from build123d import *

# Parameters (mm, degrees)
F1_DEPTH = 7.9375
F2_R     = 1.98374
F3_R     = 3.69316
F4_R     = 1.35255
F5_DEPTH = 134.38632
F6_W     = 127
F6_H     = 1.70942
F7_DEPTH = 3.175
F8_R     = 1.35255
F9_DEPTH = 1.70942
F10_R    = 0.762


with BuildPart() as f1:
    # F0 (on Top) → F1 (new body)
    with BuildSketch(Plane.XY):
        Polygon((0, 30.55874), (0, 0), (-130.96748, 0), (-130.96748, 30.55874), (-132.6769, 30.55874), (-132.6769, -1.70942), (1.70942, -1.70942), (1.70942, 30.55874), align=None)
    extrude(amount=F1_DEPTH)

    # F2
    f2_edges = [f1.edges().sort_by_distance(p)[0] for p in [
        (0, 0, 3.96875),
        (-130.96748, 0, 3.96875),
    ]]
    fillet(f2_edges, radius=F2_R)

    # F3
    f3_edges = [f1.edges().sort_by_distance(p)[0] for p in [
        (1.70942, -1.70942, 3.96875),
        (-132.6769, -1.70942, 3.96875),
    ]]
    fillet(f3_edges, radius=F3_R)

    # F4 (on face) → F5 (cut, through all)
    with BuildSketch(Plane(origin=(-132.6769, 0, 0), x_dir=(0, -1, 0), z_dir=(-1, 0, 0))):
        with Locations((-26.58999, 3.96875)):
            Circle(F4_R)
        with Locations((-5.95249, 3.96875)):
            Circle(F4_R)
    extrude(amount=-F5_DEPTH, mode=Mode.SUBTRACT)

    # F6 (on face) → F7 (join)
    with BuildSketch(Plane(origin=(0, 0, 0), x_dir=(1, 0, 0), z_dir=(0, 0, -1))):
        with Locations((-65.48374, 0.85471)):
            Rectangle(F6_W, F6_H)
    extrude(amount=F7_DEPTH)

    # F8 (on face) → F9 (cut, through all)
    with BuildSketch(Plane.XZ.offset(1.70942)):
        with Locations((-125.01499, 0.79375)):
            Circle(F8_R)
        with Locations((-65.48374, 0.79375)):
            Circle(F8_R)
        with Locations((-5.95249, 0.79375)):
            Circle(F8_R)
    extrude(amount=-F9_DEPTH, mode=Mode.SUBTRACT)

    # F10
    f10_edges = [f1.edges().sort_by_distance(p)[0] for p in [
        (0.85471, 30.55874, 0),
        (0.85471, 30.55874, 7.9375),
        (-131.82219, 30.55874, 0),
        (-131.82219, 30.55874, 7.9375),
        (-128.98374, -0.85471, -3.175),
        (-1.98374, -0.85471, -3.175),
    ]]
    fillet(f10_edges, radius=F10_R)


solid = f1.part
Source: CAD feature listing. Evaluate the final solid. Frame: model axes, mm. A direction names the side the tool comes from. Coordinates: 2 decimals unless noted, no trailing zeros. Loops run counter-clockwise (first coordinate to the right, second up) from the corner with the lowest first, then second, coordinate; pieces in that order, holes last. Notation, with made-up numbers: (-18, 5.5) - (28, 5.5) arc R27 ccw to (28, 21.5) - close; hole circle Ø2 at (-36.5, -3). An arc over 180 degrees is marked (long way). One line per item, written item: value. Start each with the question number.
1. Ray query, L1, parallel to X at y = 19.5, z = 6; L2, parallel to Y at x = -77, z = 1.25. Return the intervals inside material, ascending.
2. Section A-A (x = -10.5). Return the cut outline in (y, z) (1 decimal).
3. Contact query for flat-ended pins moving along their axis: P1, Ø1, axis at x = -54.5, z = 6, coming from the +Y side; P2, Ø4.5, axis at x = -125.01, z = 0.79, coming from the -Y side; P3, Ø0.5, axis at y = -1, z = -0.5, coming from the +X side; P4, Ø0.5, axis at y = -1, z = -0.5, coming from the -X side. Output: stop coordinate, or through.
4. Set-up query: faces 1 (the flat face through (0, 16, 4)), 2 (the cylindrical face through (0.84, 27.94, 4.03)). Return all of +Z, -Z, +X, -X, +Y, -Y with unobstructed straight access to the full face (end or side cutting, diameter ignored); none if empty.
5. Mould query, pull axis X, two halves, no side actions, for faces 3 (the cylindrical face through (0.656, -0.599, 4.024)), 4 (the flat face through (1, 14, 0)), 5 (the cylindrical face through (-123.725, -0.867, 1.2)). Classes: pulls with the +X half, pulls with the -X half, needs draft (parallel to the pull), parting line crosses it, or undercut.
Verdict:
1. L1: x = -132.68 to -130.97, 0 to 1.71
1. L2: y = -1.71 to 0
2. outline: (-1.7, -3.2) - (0, -3.2) - (0, 7.9) - (-1.7, 7.9) - close
3. P1: stops at y = 0
3. P2: stops at y = -1.71
3. P3: stops at x = -1.98
3. P4: stops at x = -128.98
4. face 1: +Z, -Z, +Y
4. face 2: +X, -X
5. face 3: pulls with the +X half
5. face 4: needs draft
5. face 5: undercut
